from build123d import *

# Parameters (mm, degrees)
F1_DEPTH = 20
F3_DEPTH = 3
F4_R     = 3
F5_R     = 3


with BuildPart() as f1:
    # F0 (on Top) → F1 (new body)
    with BuildSketch(Plane.XY):
        with BuildLine():
            Line((-17.5, -22.5), (17.5, -22.5))
            ThreePointArc((17.5, -22.5), (21.035534, -21.035534), (22.5, -17.5))
            Line((22.5, -17.5), (22.5, 17.5))
            ThreePointArc((22.5, 17.5), (21.035534, 21.035534), (17.5, 22.5))
            Line((17.5, 22.5), (-17.5, 22.5))
            ThreePointArc((-17.5, 22.5), (-21.035534, 21.035534), (-22.5, 17.5))
            Line((-22.5, 17.5), (-22.5, -17.5))
            ThreePointArc((-22.5, -17.5), (-21.035534, -21.035534), (-17.5, -22.5))
        make_face()
        with BuildLine():
            ThreePointArc((-16.7, -21.7), (-20.235534, -20.235534), (-21.7, -16.7))
            Line((-21.7, -16.7), (-21.7, 16.7))
            ThreePointArc((-21.7, 16.7), (-20.235534, 20.235534), (-16.7, 21.7))
            Line((-16.7, 21.7), (16.7, 21.7))
            ThreePointArc((16.7, 21.7), (20.235534, 20.235534), (21.7, 16.7))
            Line((21.7, 16.7), (21.7, -16.7))
            ThreePointArc((21.7, -16.7), (20.235534, -20.235534), (16.7, -21.7))
            Line((16.7, -21.7), (-16.7, -21.7))
        make_face(mode=Mode.SUBTRACT)
    extrude(amount=F1_DEPTH)

    # F2 (on Top) → F3 (join)
    with BuildSketch(Plane.XY):
        with BuildLine():
            ThreePointArc((22.5, 17.5), (21.035534, 21.035534), (17.5, 22.5))
            Line((17.5, 22.5), (-17.5, 22.5))
            ThreePointArc((-17.5, 22.5), (-21.035534, 21.035534), (-22.5, 17.5))
            Line((-22.5, 17.5), (-22.5, -17.5))
            ThreePointArc((-22.5, -17.5), (-21.035534, -21.035534), (-17.5, -22.5))
            Line((-17.5, -22.5), (17.5, -22.5))
            ThreePointArc((17.5, -22.5), (21.035534, -21.035534), (22.5, -17.5))
            Line((22.5, -17.5), (22.5, 17.5))
        make_face()
    extrude(amount=-F3_DEPTH)

    # F4
    f4_edges = [f1.edges().sort_by_distance(p)[0] for p in [
        (22.5, 0, -3),
        (21.035534, 21.035534, -3),
        (0, 22.5, -3),
        (-21.035534, 21.035534, -3),
        (-22.5, 0, -3),
        (-21.035534, -21.035534, -3),
        (0, -22.5, -3),
        (21.035534, -21.035534, -3),
    ]]
    fillet(f4_edges, radius=F4_R)

    # F5
    f5_edges = [f1.edges().sort_by_distance(p)[0] for p in [
        (0, -21.7, 0),
        (-20.235534, -20.235534, 0),
        (-21.7, 0, 0),
        (-20.235534, 20.235534, 0),
        (0, 21.7, 0),
        (20.235534, 20.235534, 0),
        (21.7, 0, 0),
        (20.235534, -20.235534, 0),
    ]]
    fillet(f5_edges, radius=F5_R)


solid = f1.part
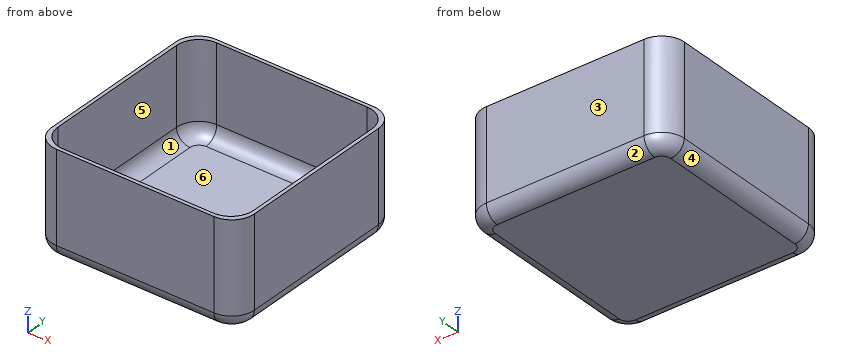
Design review of the part built by this model. Coordinates are the model's own, in mm. Face numbers are marked on the shaded views. A direction names the side the tool comes from. Give positions to 0.01 mm unless a question says otherwise; leave off trailing zeros. Write each loop counter-clockwise with the first axis right and the second up, starting at its lowest first coordinate (ties: lowest second). Pieces come first, ordered by that corner, then holes. Notation, with made-up numbers: M 25,19 L 44,19 A6 ccw 44,26 Z; hole C -30,17 d3. An arc over 180 degrees is marked long. Answer as a JSON object with one key per item and string values. Group by question number.
1) Mouldability with a two-part tool opening along X and no side actions: class the marked faces 3, 4, 5 and 6 as released by +X, released by -X, zero draft, split by the parting line, or undercut.
2) We need section B-B (y = -14.5). Give the boundary of the cut face in (x, z).
3) We need section A-A (z = 9.75). Give the boundary of the cut face in (x, y).
4) Tool access review of the marked faces 1 and 2: name each direction out of +Z, -Z, +X, -X, +Y, -Y from which nothing blocks a thin tool from reaching the whole face with its end or side.
5) For line 1 along X through (y, z) = (-16, 12.25); line 2 along Z through (x, y) = (-14, -4), list the stretches that pass through material, from the lowest coordinate up.
6) Clearance check with a flat-ended pin moving along its axis: pin 1 Ø6 at (x, y) = (-2.5, -16.5) entering from +Z. State where the tip first meets the part, or that it passes through.
Answer key:
{
 "1": {"face 3": "zero draft", "face 4": "released by -X", "face 5": "undercut", "face 6": "undercut"},
 "2": {"outline": "M -22.5,0 A3 ccw -19.5,-3 L 19.5,-3 A3 ccw 22.5,0 L 22.5,20 L 21.7,20 L 21.7,3 A3 cw 18.7,0 L -18.7,0 A3 cw -21.7,3 L -21.7,20 L -22.5,20 Z"},
 "3": {"outline": "M -22.5,-17.5 A5 ccw -17.5,-22.5 L 17.5,-22.5 A5 ccw 22.5,-17.5 L 22.5,17.5 A5 ccw 17.5,22.5 L -17.5,22.5 A5 ccw -22.5,17.5 Z; hole M -21.7,-16.7 A5 ccw -16.7,-21.7 L 16.7,-21.7 A5 ccw 21.7,-16.7 L 21.7,16.7 A5 ccw 16.7,21.7 L -16.7,21.7 A5 ccw -21.7,16.7 Z"},
 "4": {"face 1": "+Z", "face 2": "-Z, +X, -X, +Y"},
 "5": {"line 1": "x = -22.5 to -21.7, 21.7 to 22.5", "line 2": "z = -3 to 0"},
 "6": {"pin 1": "stops at z = 0.11"}
}
